Model file for the job. Use its own axes, mm. A direction names the side the tool comes from. Coordinates: 2 decimals unless noted, no trailing zeros. Write each loop counter-clockwise with the first axis right and the second up, starting at its lowest first coordinate (ties: lowest second). Pieces come first, ordered by that corner, then holes.
Q1. Pull direction X, two halves, no side cores. Call faces 1 (the flat face through (0, -25, -101)), 2 (the flat face through (0, -16, -110)), 3 (the flat face through (20.5, -7, -65)), 4 (the flat face through (0, -25, -72)): released by +X, released by -X, zero draft, split by the parting line, or undercut.
Q2. Band-saw the part on B-B, the plane x = 11. Write the cut outline in (y, z), plus the area to 3 significant figures.
Q3. Which spindle directions (+Z, -Z, +X, -X, +Y, -Y) get a long thin tool onto all of the face, cutting with end or side? Do faces 5 (the flat face through (6, -29, -87)), 6 (the flat face through (0, 11, -57)), 7 (the flat face through (0, -21, -28)), 8 (the flat face through (18, 0, -21)), 9 (the cylindrical face through (-2.752, 8.923, 1.172)). Say none if no direction does.
Q4. Band-saw the part on A-A, the plane y = -5. Write the cut outline in (x, z).
Q5. Pin check, flat tips, straight feed: P1, Ø2, axis at x = 7, z = -60, coming from the -Y side; P2, Ø8, axis at x = 11, y = -13.5, coming from the +Z side; P3, Ø1, axis at x = -4, z = -61, coming from the -Y side. Stop position of each tip, or through.
Q6. Band-saw the part on C-C, the plane y = -17. Write the cut outline in (x, z), plus the area to 3 significant figures.
Q7. Drill centre lines: probe 1 along Y at (x, z) = (6, 0); probe 2 along X at (y, z) = (10.5, 11); probe 3 along Z at (x, y) = (-1, -16). Where is each one in solid material? Low to high.
Q8. Band-saw the part on D-D, the plane y = -23. Write the cut outline in (x, z).
from build123d import *

# Parameters (mm, degrees)
SKETCH2_R           = 9
BOSS_EXTRUDE1_DEPTH = 20.5
SKETCH3_W           = 5
SKETCH3_H           = 21
CUT_EXTRUDE1_DEPTH  = 124.81134843
SKETCH4_W           = 12
SKETCH4_H           = 7
CUT_EXTRUDE2_DEPTH  = 137.401063046
CHAMFER2_SIZE       = 3


with BuildPart() as part:
    # Sketch2 → Boss-Extrude1 (new, symmetric)
    with BuildSketch(Plane(origin=(0, 0, 0), x_dir=(0, 0, -1), z_dir=(1, 0, 0))):
        with BuildLine():
            Line((0, 21), (50, 21))
            Line((50, 21), (64.704358302, 0))
            Line((64.704358302, 0), (110, 0))
            Line((110, 0), (110, -32))
            Line((110, -32), (65, -32))
            ThreePointArc((65, -32), (62.466324116, -24.291796068), (55.050125629, -21))
            Line((55.050125629, -21), (0, -21))
            ThreePointArc((0, -21), (-21, 0), (0, 21))
        make_face()
        Circle(SKETCH2_R, mode=Mode.SUBTRACT)
    extrude(amount=BOSS_EXTRUDE1_DEPTH, both=True)

    # Sketch3 → Cut-Extrude1 (cut, through all)
    with BuildSketch(Plane(origin=(0, 21, 0), x_dir=(1, 0, 0), z_dir=(0, 1, 0))):
        with Locations((18, -10.5)):
            Rectangle(SKETCH3_W, SKETCH3_H)
        with Locations((18, 10.5)):
            Rectangle(SKETCH3_W, SKETCH3_H)
        with BuildLine():
            ThreePointArc((0, 42), (-6, 36), (0, 30))
            Line((0, 30), (0, 42))
        make_face()
        with BuildLine():
            Line((0, 42), (0, 30))
            ThreePointArc((0, 30), (4.242640687, 31.757359313), (6, 36))
            ThreePointArc((6, 36), (4.242640687, 40.242640687), (0, 42))
        make_face()
        with BuildLine():
            ThreePointArc((6, 86), (4.242640687, 90.242640687), (0, 92))
            Line((0, 92), (0, 80))
            ThreePointArc((0, 80), (4.242640687, 81.757359313), (6, 86))
        make_face()
        with BuildLine():
            Line((0, 80), (0, 92))
            ThreePointArc((0, 92), (-6, 86), (0, 80))
        make_face()
    extrude(amount=-CUT_EXTRUDE1_DEPTH, mode=Mode.SUBTRACT)

    # Sketch4 → Cut-Extrude2 (cut, through all)
    with BuildSketch(Plane(origin=(0, 0, -110), x_dir=(-1, 0, 0), z_dir=(0, 0, -1))):
        with Locations((0, -28.5)):
            Rectangle(SKETCH4_W, SKETCH4_H)
    extrude(amount=-CUT_EXTRUDE2_DEPTH, mode=Mode.SUBTRACT)

    # Chamfer2
    chamfer2_edges = [part.edges().sort_by_distance(p)[0] for p in [
        (20.5, -16, -110),
        (20.5, 21, -35.5),
        (-20.5, -16, -110),
    ]]
    chamfer(chamfer2_edges, length=CHAMFER2_SIZE)


solid = part.part
Answer sheet:
1. face 1: undercut
1. face 2: zero draft
1. face 3: released by +X
1. face 4: undercut
2. outline: (-32, -110) - (0, -110) - (0, -64.7) - (21, -50) - (21, 0) arc R21 ccw to (-21, 0) - (-21, -55.05) arc R10 cw to (-32, -65) - close; hole circle Ø18 at (0, 0)
2. area: 4,470 mm2
3. face 5: +Z, -Z, -Y
3. face 6: -Z, +X, -X, +Y
3. face 7: +Z, +X, -X, -Y
3. face 8: +Z, +X, +Y, -Y
3. face 9: +X, -X
4. outline: (-20.5, -107) - (-17.5, -110) - (17.5, -110) - (20.5, -107) - (20.5, -21) - (15.5, -21) - (15.5, -7.48) - (-20.5, -7.48) - close; (-20.5, 7.48) - (15.5, 7.48) - (15.5, 20.4) - (-20.5, 20.4) - close; hole circle Ø12 at (0, -86); hole circle Ø12 at (0, -36)
5. P1: stops at y = -22.96
5. P2: stops at z = 18.73
5. P3: stops at y = -23.36
6. outline: (-20.5, -107) - (-17.5, -110) - (17.5, -110) - (20.5, -107) - (20.5, -21) - (15.5, -21) - (15.5, 12.33) - (-20.5, 12.33) - close; hole circle Ø12 at (0, -86); hole circle Ø12 at (0, -36)
6. area: 4,610 mm2
7. probe 1: y = -21 to -9, 9 to 21
7. probe 2: x = -20.5 to 15.5
7. probe 3: z = -110 to -91.92, -80.08 to -41.92, -30.08 to 13.6
8. outline: (-20.5, -107) - (-17.5, -110) - (17.5, -110) - (20.5, -107) - (20.5, -61.05) - (-20.5, -61.05) - close; hole circle Ø12 at (0, -86)
